from build123d import *

# Parameters (mm, degrees)
POCKET_DEPTH    = 8
SKETCH003_R     = 4.25
POCKET001_DEPTH = 64.001
SKETCH004_R     = 11
POCKET002_DEPTH = 8
FILLET_R        = 2
FILLET001_R     = 5


with BuildPart() as part:
    # Sketch → Revolution (revolve)
    with BuildSketch(Plane.XZ):
        Polygon((0, 0), (22.5, 0), (25, 64), (0, 64), align=None)
    revolve(axis=Axis((0, 0, 0), (0, 0, 1)))

    # Sketch002 (on Face1 of Revolution) → Pocket (cut)
    with BuildSketch(Plane(origin=(0, 0, 0), x_dir=(1, 0, 0), z_dir=(0, 0, -1))):
        Polygon((7.75, 0), (3.875, 6.711697), (-3.875, 6.711697), (-7.75, 0), (-3.875, -6.711697), (3.875, -6.711697), align=None)
    extrude(amount=-POCKET_DEPTH, mode=Mode.SUBTRACT)

    # Sketch003 (on Face1 of Pocket) → Pocket001 (cut, through all)
    with BuildSketch(Plane(origin=(0, 0, 0), x_dir=(1, 0, 0), z_dir=(0, 0, -1))):
        Circle(SKETCH003_R)
    extrude(amount=-POCKET001_DEPTH, mode=Mode.SUBTRACT)

    # Sketch004 (on Face9 of Pocket001) → Pocket002 (cut)
    with BuildSketch(Plane(origin=(0, 0, 64), x_dir=(-1, 0, 0), z_dir=(0, 0, 1))):
        Circle(SKETCH004_R)
    extrude(amount=-POCKET002_DEPTH, mode=Mode.SUBTRACT)

    # Fillet
    fillet_edges = [part.edges().sort_by_distance(p)[0] for p in [
        (-25, 0, 64),
        (11, 0, 64),
    ]]
    fillet(fillet_edges, radius=FILLET_R)

    # Fillet001
    fillet001_edges = [part.edges().sort_by_distance(p)[0] for p in [
        (-22.5, 0, 0),
    ]]
    fillet(fillet001_edges, radius=FILLET001_R)


solid = part.part
Input: part model. Units: mm. Frame: model coordinates. A direction names the side the tool comes from. Give positions to 0.01 mm unless a question says otherwise; leave off trailing zeros. Loops run counter-clockwise (first coordinate to the right, second up) from the corner with the lowest first, then second, coordinate; pieces in that order, holes last. Notation, with made-up numbers: M 13,84.25 L 35,84.25 A16 cw 35,91.25 Z; hole C 79.25,-37 d9. An arc over 180 degrees is marked long. Use one line per item in the form item = value.
1. Section query B-B, the plane z = 30.5. Return the cut outline in (x, y), and give its area (3 significant figures).
Numbers:
outline = C 0,0 d47.38; hole C 0,0 d8.5
area = 1,710 mm²
2. First-contact query: pin 1 (10 mm diameter, centred on x = 9, z = 46, fed in from +Y); pin 2 (8 mm diameter, centred on x = -6.5, z = 9.5, fed in from -Y); pin 3 (10 mm diameter, centred on y = -4, z = 56, fed in from -X); pin 4 (7.5 mm diameter, centred on x = 0, y = 0, fed in from +Z). Flat tips, straight axial feed; report the tip coordinate or a pass-through.
Numbers:
pin_1 = 23.99
pin_2 = -22.76
pin_3 = -24.82
pin_4 = through
3. Section query C-C, the plane z = 15. Return the cut outline in (x, y), and give its area (3 significant figures).
Numbers:
outline = C 0,0 d46.17; hole C 0,0 d8.5
area = 1,620 mm²
4. Section query A-A, the plane x = 0. Return the cut outline in (y, z).
Numbers:
outline = M -24.92,61.92 L -22.69,4.8 A5 ccw -17.69,0 L -6.71,0 L -6.71,8 L -4.25,8 L -4.25,56 L -11,56 L -11,62 A2 ccw -13,64 L -22.92,64 A2 ccw Z; M 4.25,8 L 6.71,8 L 6.71,0 L 17.69,0 A5 ccw 22.69,4.8 L 24.92,61.92 A2 ccw 22.92,64 L 13,64 A2 ccw 11,62 L 11,56 L 4.25,56 Z
5. Pull-direction query (Y, two-part tool) for faces 4 (the face through (0, 5, 56)), 5 (the face through (22.72, 7.15, 33.76)), 6 (the face through (0, -8, 0)); classes: released by +Y, released by -Y, zero draft, split by the parting line, or undercut.
Numbers:
face_4 = undercut
face_5 = split by the parting line
face_6 = zero draft
6. Line query: L1, parallel to X at y = 0, z = 35; L2, parallel to Y at x = 0, z = 58; L3, parallel to Y at x = 0, z = 60.3. Output: solid intervals per line, ascending.
Numbers:
L1 = -23.87 to -4.25, 4.25 to 23.87
L2 = -24.77 to -11, 11 to 24.77
L3 = -24.86 to -11, 11 to 24.86
7. Reachability of faces 1 (the face through (10, -10, 64)), 2 (the face through (3.3, -3.1, 8)), 3 (the face through (2.38, 10.74, 59.04)) from +Z, -Z, +X, -X, +Y, -Y: full face, straight path, thin tool, end or side. Return the list, or none.
Numbers:
face_1 = +Z, +X, -X, +Y, -Y
face_2 = -Z
face_3 = +Z
